Part model, mm, in its own coordinate system. Coordinates: 2 decimals unless noted, no trailing zeros. Answer as CSV lines item,"result".
from build123d import *

# Parameters (mm, degrees)
PROFILE_SKETCH_R      = 2.1
PROFILE_EXTRUDE_DEPTH = 475


with BuildPart() as part:
    # Profile Sketch → Profile Extrude (new body)
    with BuildSketch(Plane(origin=(0, 0, 0), x_dir=(0, 0, -1), z_dir=(1, 0, 0))):
        with BuildLine():
            Line((5.42, 10), (-5.42, 10))
            Line((-5.42, 10), (-6.875, 8.545))
            Line((-6.875, 8.545), (-6.875, 8.2))
            Line((-6.875, 8.2), (-4.5, 8.2))
            Line((-4.5, 8.2), (-4.5, 6.56))
            Line((-4.5, 6.56), (-7.16, 3.9))
            Line((-7.16, 3.9), (-9.79, 3.9))
            Line((-9.79, 3.9), (-10, 3.69))
            Line((-10, 3.69), (-10.21, 3.9))
            Line((-10.21, 3.9), (-12.84, 3.9))
            Line((-12.84, 3.9), (-15.5, 6.56))
            Line((-15.5, 6.56), (-15.5, 8.2))
            Line((-15.5, 8.2), (-13.125, 8.2))
            Line((-13.125, 8.2), (-13.125, 8.545))
            Line((-13.125, 8.545), (-14.58, 10))
            Line((-14.58, 10), (-19.5, 10))
            ThreePointArc((-19.5, 10), (-19.853553391, 9.853553391), (-20, 9.5))
            Line((-20, 9.5), (-20, 4.58))
            Line((-20, 4.58), (-18.545, 3.125))
            Line((-18.545, 3.125), (-18.2, 3.125))
            Line((-18.2, 3.125), (-18.2, 5.5))
            Line((-18.2, 5.5), (-16.56, 5.5))
            Line((-16.56, 5.5), (-13.9, 2.838679656))
            Line((-13.9, 2.838679656), (-13.9, 0.21))
            Line((-13.9, 0.21), (-13.69, 0))
            Line((-13.69, 0), (-13.9, -0.21))
            Line((-13.9, -0.21), (-13.9, -2.838679656))
            Line((-13.9, -2.838679656), (-16.56, -5.5))
            Line((-16.56, -5.5), (-18.2, -5.5))
            Line((-18.2, -5.5), (-18.2, -3.125))
            Line((-18.2, -3.125), (-18.545, -3.125))
            Line((-18.545, -3.125), (-20, -4.58))
            Line((-20, -4.58), (-20, -9.5))
            ThreePointArc((-20, -9.5), (-19.853553391, -9.853553391), (-19.5, -10))
            Line((-19.5, -10), (-14.58, -10))
            Line((-14.58, -10), (-13.125, -8.545))
            Line((-13.125, -8.545), (-13.125, -8.2))
            Line((-13.125, -8.2), (-15.5, -8.2))
            Line((-15.5, -8.2), (-15.5, -6.56))
            Line((-15.5, -6.56), (-12.84, -3.9))
            Line((-12.84, -3.9), (-10.21, -3.9))
            Line((-10.21, -3.9), (-10, -3.69))
            Line((-10, -3.69), (-9.79, -3.9))
            Line((-9.79, -3.9), (-7.16, -3.9))
            Line((-7.16, -3.9), (-4.5, -6.56))
            Line((-4.5, -6.56), (-4.5, -8.2))
            Line((-4.5, -8.2), (-6.875, -8.2))
            Line((-6.875, -8.2), (-6.875, -8.545))
            Line((-6.875, -8.545), (-5.42, -10))
            Line((-5.42, -10), (5.42, -10))
            Line((5.42, -10), (6.875, -8.545))
            Line((6.875, -8.545), (6.875, -8.2))
            Line((6.875, -8.2), (4.5, -8.2))
            Line((4.5, -8.2), (4.5, -6.56))
            Line((4.5, -6.56), (7.16, -3.9))
            Line((7.16, -3.9), (9.79, -3.9))
            Line((9.79, -3.9), (10, -3.69))
            Line((10, -3.69), (10.21, -3.9))
            Line((10.21, -3.9), (12.84, -3.9))
            Line((12.84, -3.9), (15.5, -6.56))
            Line((15.5, -6.56), (15.5, -8.2))
            Line((15.5, -8.2), (13.125, -8.2))
            Line((13.125, -8.2), (13.125, -8.545))
            Line((13.125, -8.545), (14.58, -10))
            Line((14.58, -10), (19.5, -10))
            ThreePointArc((19.5, -10), (19.853553391, -9.853553391), (20, -9.5))
            Line((20, -9.5), (20, -4.58))
            Line((20, -4.58), (18.545, -3.125))
            Line((18.545, -3.125), (18.2, -3.125))
            Line((18.2, -3.125), (18.2, -5.5))
            Line((18.2, -5.5), (16.56, -5.5))
            Line((16.56, -5.5), (13.9, -2.838679656))
            Line((13.9, -2.838679656), (13.9, -0.21))
            Line((13.9, -0.21), (13.69, 0))
            Line((13.69, 0), (13.9, 0.21))
            Line((13.9, 0.21), (13.9, 2.838679656))
            Line((13.9, 2.838679656), (16.56, 5.5))
            Line((16.56, 5.5), (18.2, 5.5))
            Line((18.2, 5.5), (18.2, 3.125))
            Line((18.2, 3.125), (18.545, 3.125))
            Line((18.545, 3.125), (20, 4.58))
            Line((20, 4.58), (20, 9.5))
            ThreePointArc((20, 9.5), (19.853553391, 9.853553391), (19.5, 10))
            Line((19.5, 10), (14.58, 10))
            Line((14.58, 10), (13.125, 8.545))
            Line((13.125, 8.545), (13.125, 8.2))
            Line((13.125, 8.2), (15.5, 8.2))
            Line((15.5, 8.2), (15.5, 6.56))
            Line((15.5, 6.56), (12.84, 3.9))
            Line((12.84, 3.9), (10.21, 3.9))
            Line((10.21, 3.9), (10, 3.69))
            Line((10, 3.69), (9.79, 3.9))
            Line((9.79, 3.9), (7.16, 3.9))
            Line((7.16, 3.9), (4.5, 6.56))
            Line((4.5, 6.56), (4.5, 8.2))
            Line((4.5, 8.2), (6.875, 8.2))
            Line((6.875, 8.2), (6.875, 8.545))
            Line((6.875, 8.545), (5.42, 10))
        make_face()
        with Locations(Location((-10, 0, 0), (0, 0, 180))):
            Circle(PROFILE_SKETCH_R, mode=Mode.SUBTRACT)
        with Locations(Location((10, 0, 0), (0, 0, 180))):
            Circle(PROFILE_SKETCH_R, mode=Mode.SUBTRACT)
        Polygon((2.7, 8.2), (-2.7, 8.2), (-2.7, 6.238679656), (-6.1, 2.838679656), (-6.1, -0.21), (-6.1, -2.838679656), (-2.7, -6.238679656), (-2.7, -8.2), (2.7, -8.2), (2.7, -6.238679656), (6.1, -2.838679656), (6.1, -0.21), (6.1, 2.838679656), (2.7, 6.238679656), align=None, mode=Mode.SUBTRACT)
    extrude(amount=PROFILE_EXTRUDE_DEPTH)


solid = part.part
Q1. Wall check: L1, parallel to Z at x = 225, y = -0.5; L2, parallel to Z at x = 431, y = 7.25; L3, parallel to Y at x = 200.5, z = 10. Give the ranges that are in metal, low to high.
Results:
L1,"z = -13.9 to -12.04, -7.96 to -6.1, 6.1 to 7.96, 12.04 to 13.9"
L2,"z = -20 to -15.5, -4.5 to -2.7, 2.7 to 4.5, 15.5 to 20"
L3,"y = -3.69 to -2.1, 2.1 to 3.69"
Q2. Saw through at A-A (x = 422). Count the separate pieces of the cut face and the enclosed holes in it, then the cut area to 3 significant figures.
Results:
separate pieces,"1"
enclosed holes,"3"
area,"300 mm^2"
Q3. Flat gauge pins, fed straight in: pin 1 (1 mm diameter, centred on x = 367, y = -2, fed in from -Z); pin 2 (1.5 mm diameter, centred on x = 423.5, z = -12, fed in from +Y); pin 3 (1.2 mm diameter, centred on x = 212, y = 3.5, fed in from -Z); pin 4 (4 mm diameter, centred on y = 0, z = -10, fed in from -X). Where does each tip first touch, or does it go through?
Results:
pin 1,"stops at z = -13.9"
pin 2,"stops at y = 3.9"
pin 3,"stops at z = -19.52"
pin 4,"passes through"
